Can you work these out from the model? Positions are in its coordinate system, mm. Face numbers are marked on the shaded views. A direction names the side the tool comes from. Give positions to 0.01 mm unless a question says otherwise; leave off trailing zeros. Write each loop counter-clockwise with the first axis right and the second up, starting at its lowest first coordinate (ties: lowest second). Pieces come first, ordered by that corner, then holes. Notation, with made-up numbers: M 37.25,-1.5 L 52.25,-1.5 A10 ccw 52.25,4.5 Z; hole C 37.25,-29.5 d6. An arc over 180 degrees is marked long. Write each question's results on one line, items separated by ' | '.
Autodesk Inventor part; units mm, degrees
ref_plane "Work Plane1" through (1.525, 0, 0) normal (0, 0, 1) x (1, 0, 0)
ref_plane "YZ Plane" through (0, 0, 0) normal (1, 0, 0) x (0, 1, 0)
ref_plane "XZ Plane" through (0, 0, 0) normal (0, 1, 0) x (-1, 0, 0)
sketch "Sketch1" plane through (0, 0, 0) normal (0, 0, 1) x (1, 0, 0)
  line L0 (0, 5.5626) -> (0, 3.302)
  line L1 (3.175, 3.175) -> (19.05, 3.175)
  line L2 (19.05, 3.175) -> (19.05, 0)
  line L3 (19.05, 0) -> (-0.0001, 0)
  line L4 (-3.8101, 0) -> (22.86, 0)
  line L5 (-0.0001, 0) -> (-0.0001, 5.5626)
  line L6 (-0.0001, 5.5626) -> (0, 5.5626)
  line L7 (3.175, 3.175) -> (0.0019, 3.302)
  line L8 (0.0019, 3.302) -> (0, 3.302)
  line L9 (0, -1.1125) -> (0, 6.6751)
  dimension "d0" = 19.05
  dimension "d1" = 15.875
  dimension "d2" = 6.35
  dimension "d9" = 0.0001
  dimension "d10" = 11.1252
  dimension "d13" = 3.1731
  dimension "d14" = 6.604
revolve "Body" add sketch "Sketch1" angle 360 about axis through (19.05, 0, 0) along (-1, 0, 0)
sketch "Sketch2" plane through (-0.0001, 0, 0) normal (-1, 0, 0) x (0, 0, 1)
  line L0 (0, 6.4231) -> (5.5626, 3.2116)
  line L1 (5.5626, 3.2116) -> (5.5626, -3.2116)
  line L2 (5.5626, -3.2116) -> (0, -6.4231)
  line L3 (0, -6.4231) -> (-5.5626, -3.2116)
  line L4 (-5.5626, -3.2116) -> (-5.5626, 3.2116)
  line L5 (-5.5626, 3.2116) -> (0, 6.4231)
  point P0 (0, 0)
  point P1 (0, 0)
  dimension "d11" = 11.1252
extrude "Head" add sketch "Sketch2" along normal blind 4.7752
sketch "Sketch4" plane through (0, 0, 0) normal (0, 0, 1) x (1, 0, 0)
  line L0 (-4.7753, 5.5626) -> (-4.7753, 6.4231)
  line L1 (-4.7753, 6.4231) -> (-4.2785, 6.4231)
  line L2 (-4.2785, 6.4231) -> (-4.7753, 5.5626)
  line L3 (-5.7303, 0) -> (0.9549, 0)
  line L4 (-0.0001, 6.4231) -> (-4.7753, 6.4231)
  line L5 (-4.7753, 3.2116) -> (-4.7753, 6.4231)
  dimension "d5" = 30
  dimension "d19" = 11.1252
revolve "Chamfer1" cut sketch "Sketch4" angle 360 about axis through (-10, 0, 0) along (1, 0, 0)
thread "Thread"
chamfer "Chamfer2" distance 0.7791 distance2 0.7553 1 edges at (19.05, -3.175, 0) measured on face at (19.05, -0.5663, 0.5832)
ref_plane "Work Plane1" through (1.525, 0, 0) normal (0, 0, 1) x (1, 0, 0)
fillet "Fillet2" radius 0.762 1 edges at (0.0019, -3.302, 0)
equation "\"d0\" = NLG"
equation "\"d1\" = GEL"
equation "\"d2\" = GD"
equation "\"d10\" = SD2"
equation "\"d14\" = BDM"
equation "\"d11\" = SW"
equation "\"d3\" = KOH - SD"
equation "\"d5\" = ANG1"
equation "\"d19\" = SW0"
equation "\"d63\" = R"
equation "\"d15\" = GEL"
equation "\"d6\" = -0.5 * SPD + 0.5 * GD"
equation "\"NLG\" = 19.05"
equation "\"GD\" = NND"
equation "\"BDM\" = 6.604"
equation "\"KOH\" = 4.7752"
equation "\"GEL\" = 15.875"
equation "\"SW\" = 11.1252"
equation "\"SW0\" = SW"
equation "\"SPD\" = GD1"
equation "\"SD2\" = SW"
equation "\"SD\" = 0"
equation "\"ANG1\" = 30deg"
equation "\"GAL\" = 3.173"
equation "\"GUL\" = 0.238 * GAL"
equation "\"R\" = 0.762"
equation "\"d62\" = -NLG - SD + GUL"
equation "\"GD1\" = 4.79184"
equation "\"THREADDIA\" = 6.35"
equation "\"TOA\" = 30deg"
equation "\"NND\" = 6.35"
equation "\"E0\" = 1.155 * SW"
properties part number "ANSI/ASME B18.2.1 - 1/4-20 UNC - 0.75" material "Steel, Mild"
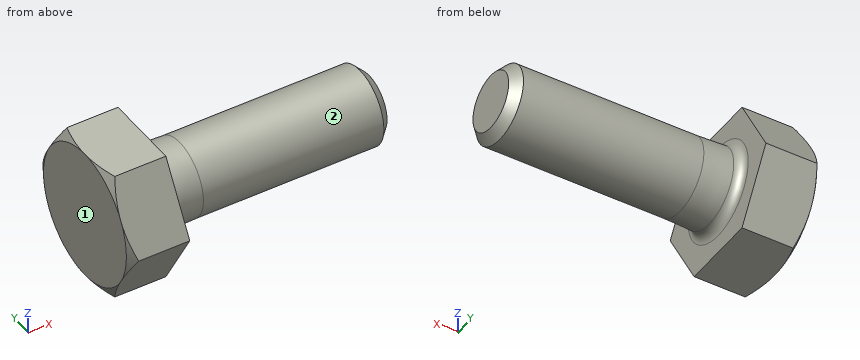
Item 1: I'm going to push flat-ended pins straight in: pin 1 (1 mm diameter, centred on x = 6, z = 1.5, fed in from +Y); pin 2 (5 mm diameter, centred on x = 9.5, y = -3, fed in from +Z); pin 3 (6 mm diameter, centred on x = 9.5, z = 2, fed in from +Y) (3 decimals); pin 4 (2 mm diameter, centred on x = 5, y = 4.5, fed in from +Z). Where does each tip first touch, or does it pass through?
Geometry says:
pin 1: stops at y = 3.01 | pin 2: stops at z = 3.14 | pin 3: stops at y = 3.175 | pin 4: passes through
Item 2: I want a section at A-A, the plane x = -1. Please give me the cut outline in (y, z), and give its area (3 significant figures).
Geometry says:
outline: M -6.42,0 L -3.21,-5.56 L 3.21,-5.56 L 6.42,0 L 3.21,5.56 L -3.21,5.56 Z | area: 107 mm2
Item 3: I want a section at B-B, the plane x = 6.25. Please give me the cut outline in (y, z) (3 decimals), and give its area (3 significant figures).
Geometry says:
outline: C 0,0 d6.35 | area: 31.7 mm2
Item 4: If I drill on line 1 (X direction, y = -1, z = -5); line 2 (Z direction, x = 2, y = -0.25); line 3 (Y direction, x = 12.5, z = 0.5), over which ranges is the centre line in solid material (lowest first)? Write a range as from..to.
Geometry says:
line 1: x = -4.78..0 | line 2: z = -3.21..3.21 | line 3: y = -3.14..3.14
Item 5: For the marked faces 1 and 2, which set-ups out of +Z, -Z, +X, -X, +Y, -Y let a thin tool reach every point of the face, with its end or its side?
Geometry says:
face 1: +Z, -Z, -X, +Y, -Y | face 2: +X
Item 6: I want a section at C-C, the plane x = 2.75. Please give me the cut outline in (y, z).
Geometry says:
outline: C 0,0 d6.38
